```python
from build123d import *

# Parameters (mm, degrees)
BOSS_EXTRUDE2_DEPTH   = 3
BOSS_EXTRUDE2_2_DEPTH = 3
SKETCH4_W             = 21
SKETCH4_H             = 23
BOSS_EXTRUDE4_DEPTH   = 0.2
SKETCH6_W             = 2
SKETCH6_H             = 4.398930514
SKETCH6_H_2           = 2.53591928
BOSS_EXTRUDE5_DEPTH   = 3.2
BOSS_EXTRUDE6_DEPTH   = 4.398930514
BOSS_EXTRUDE7_DEPTH   = 2.53591928


with BuildPart() as part:
    # Sketch1 → Boss-Extrude2 (new body)
    with BuildSketch(Plane(origin=(0, 0, 0), x_dir=(1, 0, 0), z_dir=(0, 1, 0))):
        Polygon((-10.5, -11.5), (-10.5, -6.046480624), (-8.5, -6.046480624), (-8.5, -9.5), (8.5, -9.5), (8.5, 2.051915147), (10.5, 2.051915147), (10.5, -11.5), align=None)
    extrude(amount=BOSS_EXTRUDE2_DEPTH)



with BuildPart() as body_2:
    # Sketch1 → Boss-Extrude2 2 (new body)
    with BuildSketch(Plane(origin=(0, 0, 0), x_dir=(1, 0, 0), z_dir=(0, 1, 0))):
        Polygon((-8.5, 9.5), (8.5, 9.5), (8.5, 5.587834427), (10.5, 5.587834427), (10.5, 11.5), (-10.5, 11.5), (-10.5, -0.64755011), (-8.5, -0.64755011), align=None)
    extrude(amount=BOSS_EXTRUDE2_2_DEPTH)


with BuildPart() as part_1:
    add(part.part)

    add(body_2.part)  # Boss-Extrude4 merges body 2
    # Sketch4 → Boss-Extrude4 (add)
    with BuildSketch(Plane(origin=(0, 0, 0), x_dir=(1, 0, 0), z_dir=(0, 1, 0))):
        Rectangle(SKETCH4_W, SKETCH4_H)
    extrude(amount=BOSS_EXTRUDE4_DEPTH)

    # Sketch6 → Boss-Extrude5 (add)
    with BuildSketch(Plane(origin=(0, 0.2, 0), x_dir=(1, 0, 0), z_dir=(0, 1, 0))):
        with Locations((-9.501045586, -3.347015367)):
            Rectangle(SKETCH6_W, SKETCH6_H)
        with Locations((9.496513771, 3.819874787)):
            Rectangle(SKETCH6_W, SKETCH6_H_2)
    extrude(amount=BOSS_EXTRUDE5_DEPTH)

    # Sketch7 → Boss-Extrude6 (add)
    with BuildSketch(Plane.XY.offset(5.546480624)):
        Polygon((-10.501045586, 3.4), (-10.501045586, 5.9), (-7.001045586, 3.4), align=None)
    extrude(amount=-BOSS_EXTRUDE6_DEPTH)

    # Sketch8 → Boss-Extrude7 (add)
    with BuildSketch(Plane.XY.offset(-2.551915147)):
        Polygon((10.496513771, 3.4), (10.496513771, 5.9), (6.496513771, 3.4), align=None)
    extrude(amount=-BOSS_EXTRUDE7_DEPTH)


solid = part_1.part
```
The listing builds one solid part. Answer for the finished solid, in the listing's coordinates (mm). A direction names the side the tool comes from. Coordinates: 2 decimals unless noted, no trailing zeros. Write each loop counter-clockwise with the first axis right and the second up, starting at its lowest first coordinate (ties: lowest second). Pieces come first, ordered by that corner, then holes. Notation, with made-up numbers: (-28.5, 26.5) - (-24.5, 26.5) arc R10 cw to (-24.5, 31.5) - close; hole circle Ø6 at (22.5, 73). An arc over 180 degrees is marked (long way). Return JSON: item names as keys, results as strings. Group by question number.
Q1. Find the intervals of material crossed by line 1 along Z through (x, y) = (9.25, 1.55); line 2 along Z through (x, y) = (0, 1.45); line 3 along X through (y, z) = (2.65, -7), in increasing order. Write a range as [from, to].
Q2. Flat-ended cylindrical pins translate along their axes: pin 1 Ø1.3 at (y, z) = (2, -3.5) entering from +X; pin 2 Ø2 at (y, z) = (5, -0.5) entering from +X; pin 3 Ø1.1 at (x, y) = (-9, 4) entering from +Z; pin 4 Ø9.5 at (x, z) = (-1.5, 1) entering from +Y. Find the tip coordinate at first contact, or state that the pin passes through.
Q3. For a pull along Y with two mould halves and no side action, classify faces 4 (the flat face through (9, 2, -2.052)), 5 (the flat face through (0, 0, 0)), 6 (the flat face through (8.497, 2, -4)) as +Y half, -Y half, draft (parallel to the pull), parting line (faces both ways), or undercut.
Q4. Which of the six approach directions +Z, -Z, +X, -X, +Y, -Y give full straight-line access (tool end or side, diameter ignored) to faces 1 (the flat face through (-8.501, 2, 3)), 2 (the flat face through (-8.5, 2, -4)), 3 (the flat face through (-10, 3, 5.546))?
Q5. The part is cut by section A-A on x = -8. Write down the section's boundary in (y, z), and give its area (3 significant figures).
Q6. The part is cut by section B-B on y = 4.35. Write down the section's boundary in (x, z).
Q7. The part is cut by section D-D on y = 2.5. Write down the section's boundary in (x, z).
Evaluation:
{
 "1": {"line 1": "z = [-11.5, -5.59], [-5.09, -2.55], [-2.05, 11.5]", "line 2": "z = [-11.5, -9.5], [9.5, 11.5]", "line 3": "x = [-10.5, -8.5], [8.5, 10.5]"},
 "2": {"pin 1": "stops at x = 10.5", "pin 2": "passes through", "pin 3": "stops at z = 5.55", "pin 4": "stops at y = 0.2"},
 "3": {"face 4": "draft", "face 5": "-Y half", "face 6": "undercut"},
 "4": {"face 1": "none", "face 2": "+Y", "face 3": "-X, +Y"},
 "5": {"outline": "(0, -11.5) - (3, -11.5) - (3, -9.5) - (0.2, -9.5) - (0.2, 9.5) - (3, 9.5) - (3, 11.5) - (0, 11.5) - close; (3.4, 1.15) - (4.11, 1.15) - (4.11, 5.55) - (3.4, 5.55) - close", "area": "18.9 mm2"},
 "6": {"outline": "(-10.5, 1.15) - (-8.33, 1.15) - (-8.33, 5.55) - (-10.5, 5.55) - close; (8.02, -5.09) - (10.5, -5.09) - (10.5, -2.55) - (8.02, -2.55) - close"},
 "7": {"outline": "(-10.5, -11.5) - (10.5, -11.5) - (10.5, -5.59) - (8.5, -5.59) - (8.5, -9.5) - (-8.5, -9.5) - (-8.5, 0.65) - (-10.5, 0.65) - close; (-10.5, 1.15) - (-8.5, 1.15) - (-8.5, 5.55) - (-10.5, 5.55) - close; (-10.5, 6.05) - (-8.5, 6.05) - (-8.5, 9.5) - (8.5, 9.5) - (8.5, -2.05) - (10.5, -2.05) - (10.5, 11.5) - (-10.5, 11.5) - close; (8.5, -5.09) - (10.5, -5.09) - (10.5, -2.55) - (8.5, -2.55) - close"}
}
